from build123d import *

# Parameters (mm, degrees)
F0_W     = 30
F0_H     = 10
F1_DEPTH = 5
F2_R     = 2.5
F3_DEPTH = 10
F4_R     = 1.5
F5_DEPTH = 5.001
F6_SIZE  = 1
F7_R     = 1


# Not quite as in the source:
# - a feature names something its author has since deleted; it is built from what else it names


with BuildPart() as f1:
    # F0 (on Front) → F1 (new body)
    with BuildSketch(Plane.XZ):
        with Locations((15, 10.7978725549)):
            Rectangle(F0_W, F0_H)
    extrude(amount=F1_DEPTH)

    # F2 (on face) → F3 (join)
    with BuildSketch(Plane.XZ.offset(5)):
        with Locations((10, 10.7978725549)):
            Circle(F2_R)
    extrude(amount=F3_DEPTH)

    # F4 (on face) → F5 (cut, through all)
    with BuildSketch(Plane.XZ.offset(5)):
        with Locations((22, 10.7978725549)):
            Circle(F4_R)
    extrude(amount=-F5_DEPTH, mode=Mode.SUBTRACT)

    # F6
    f6_edges = [f1.edges().sort_by_distance(p)[0] for p in [
        (15, -5, 15.797873),
    ]]
    chamfer(f6_edges, length=F6_SIZE)

    # F7
    f7_edges = [f1.edges().sort_by_distance(p)[0] for p in [
        (15, 0, 15.797873),
    ]]
    fillet(f7_edges, radius=F7_R)


solid = f1.part
Verification items for the finished model (mm, model axes). Coordinates: 2 decimals unless noted, no trailing zeros. Loops run counter-clockwise (first coordinate to the right, second up) from the corner with the lowest first, then second, coordinate; pieces in that order, holes last. Notation, with made-up numbers: M 55.5,-28 L 97.5,-28 A17 ccw 97.5,-2 Z; hole C 2,9.25 d1. An arc over 180 degrees is marked long. One line per item, written item: value.
1. Mould release check, pull along X, two halves, no side actions. Record for faces 1 (the flat face through (0, -2, 11)), 2 (the cylindrical face through (20.5, -2.54, 10.86)), 3 (the flat face through (15, -2, 5.798)), 4 (the cylindrical face through (9.458, -9.93, 8.357)): pulls with the +X half, pulls with the -X half, needs draft (parallel to the pull), parting line crosses it, or undercut.
Answers follow:
face 1: pulls with the -X half
face 2: undercut
face 3: needs draft
face 4: parting line crosses it
2. Section check B-B on x = 10. Record the cut outline in (y, z), plus the area to 3 significant figures.
Answers follow:
outline: M -15,8.3 L -5,8.3 L -5,5.8 L 0,5.8 L 0,14.8 A1 ccw -1,15.8 L -4,15.8 L -5,14.8 L -5,13.3 L -15,13.3 Z
area: 99.3 mm^2
3. Section check C-C on y = -2.5. Record the cut outline in (x, z).
Answers follow:
outline: M 0,5.8 L 30,5.8 L 30,15.8 L 0,15.8 Z; hole C 22,10.8 d3
4. Section check A-A on x = 22. Record the cut outline in (y, z), plus the area to 3 significant figures.
Answers follow:
outline: M -5,5.8 L 0,5.8 L 0,9.3 L -5,9.3 Z; M -5,12.3 L 0,12.3 L 0,14.8 A1 ccw -1,15.8 L -4,15.8 L -5,14.8 Z
area: 34.3 mm^2
5. Gauge pin test, flat ends, axial feed: P1, Ø1.5, axis at y = -11.5, z = 14.5, coming from the -X side; P2, Ø1.5, axis at y = -9, z = 11, coming from the +X side; P3, Ø4, axis at x = 7.5, y = -12.5, coming from the -Z side. Record the tip position at first contact, or that the pin passes through.
Answers follow:
P1: through
P2: x = 12.5
P3: z = 8.35
6. Section check D-D on z = 6.5. Record the cut outline in (x, y).
Answers follow:
outline: M 0,-5 L 30,-5 L 30,0 L 0,0 Z
7. Material ranges on line 1 along Z through (x, y) = (22, -1.5); line 2 along Y through (x, z) = (8.25, 6.5); line 3 along X through (y, z) = (-3.25, 10.5), recorded low to high. Write a range as from..to.
Answers follow:
line 1: 5.8..9.3, 12.3..15.8
line 2: -5..0
line 3: 0..20.53, 23.47..30
